Check sheet for the modelled part. Datum: model origin and axes. Units: mm. Face numbers are marked on the shaded views. A direction names the side the tool comes from. Round coordinates to 2 decimals unless told otherwise and drop trailing zeros. Write each loop counter-clockwise with the first axis right and the second up, starting at its lowest first coordinate (ties: lowest second). Pieces come first, ordered by that corner, then holes.
Item 1: Tool access check on the marked faces 1, 2, 3 and 4. Record the directions out of +Z, -Z, +X, -X, +Y, -Y that give a thin tool (end or side, any length) a straight path to the whole face; none if there is none.
Item 2: Cross-section at D-D on y = 4. Enter the section's corners in (x, z).
Item 3: Go/stop test with flat-tipped pins: pin 1 Ø1.5 at (x, z) = (6.5, 2) entering from -Y; pin 2 Ø2 at (x, y) = (8, 0) entering from -Z; pin 3 Ø2 at (x, z) = (10.5, -2.5) entering from -Y; pin 4 Ø4 at (y, z) = (-3.5, 5) entering from +X. Record where each tip stops, or that it passes through.
Item 4: Cross-section at C-C on x = -4.5. Enter the section's corners in (y, z), plus the area to 3 significant figures.
Item 5: Cross-section at B-B on z = 1.5. Enter the section's corners in (x, y).
Item 6: Material ranges on line 1 (X direction, y = -4, z = 3.5); line 2 (X direction, y = -1.5, z = -3.5); line 3 (Z direction, x = -6, y = -1.5), recorded low to high.
from build123d import *

# Parameters (mm, degrees)
SKETCH_1_R          = 3.5
EXTRUDE_1_DEPTH     = 7.3
SKETCH_2_R          = 5
EXTRUDE_2_DEPTH     = 4.1
SKETCH_3_R          = 5
EXTRUDE_3_DEPTH     = 4.1
EXTRUDE_START       = 6
SKETCH_4_R          = 3.5
EXTRUDE_4_DEPTH     = 6
CUT_EXTRUDE_START   = -3.2
CUT_EXTRUDE_1_DEPTH = 3.2


with BuildPart() as part:
    # 草图1 → 凸台-拉伸1 (new body)
    with BuildSketch(Plane(origin=(0, 0, 0), x_dir=(0, 0, -1), z_dir=(1, 0, 0))):
        Circle(SKETCH_1_R)
    extrude(amount=-EXTRUDE_1_DEPTH)

    # 草图2 → 凸台-拉伸2 (add)
    with BuildSketch(Plane(origin=(0, 0, 0), x_dir=(0, 0, -1), z_dir=(1, 0, 0))):
        with Locations((1.49, 0)):
            Circle(SKETCH_2_R)
    extrude(amount=EXTRUDE_2_DEPTH)

    # 草图3 → 凸台-拉伸3 (add)
    with BuildSketch(Plane(origin=(4.1, 0, 0), x_dir=(0, 0, -1), z_dir=(1, 0, 0))):
        with Locations(Location((-1.49, 0, 0), (0, 0, 287.337518018))):
            Circle(SKETCH_3_R)
    extrude(amount=EXTRUDE_3_DEPTH)

    # 草图4 → 凸台-拉伸4 (add)
    with BuildSketch(Plane(origin=(8.2, 0, 0), x_dir=(0, 0, -1), z_dir=(1, 0, 0)).offset(EXTRUDE_START)):
        Circle(SKETCH_4_R)
    extrude(amount=-EXTRUDE_4_DEPTH)

    # 草图7 → 切除-拉伸1 (cut)
    with BuildSketch(Plane.ZY.offset(7.3).offset(CUT_EXTRUDE_START)):
        with BuildLine():
            Line((-2.5, 0), (-3.5, 0))
            ThreePointArc((-3.5, 0), (-3.240370349, -1.322875656), (-2.5, -2.449489743))
            Line((-2.5, -2.449489743), (-2.5, 0))
        make_face()
        with BuildLine():
            ThreePointArc((-2.5, 2.449489743), (-3.240370349, 1.322875656), (-3.5, 0))
            Line((-3.5, 0), (-2.5, 0))
            Line((-2.5, 0), (-2.5, 2.449489743))
        make_face()
        with BuildLine():
            Line((2.5, 0), (2.5, -2.449489743))
            ThreePointArc((2.5, -2.449489743), (3.240370349, -1.322875656), (3.5, 0))
            Line((3.5, 0), (2.5, 0))
        make_face()
        with BuildLine():
            ThreePointArc((3.5, 0), (3.240370349, 1.322875656), (2.5, 2.449489743))
            Line((2.5, 2.449489743), (2.5, 0))
            Line((2.5, 0), (3.5, 0))
        make_face()
    extrude(amount=CUT_EXTRUDE_1_DEPTH, mode=Mode.SUBTRACT)


solid = part.part
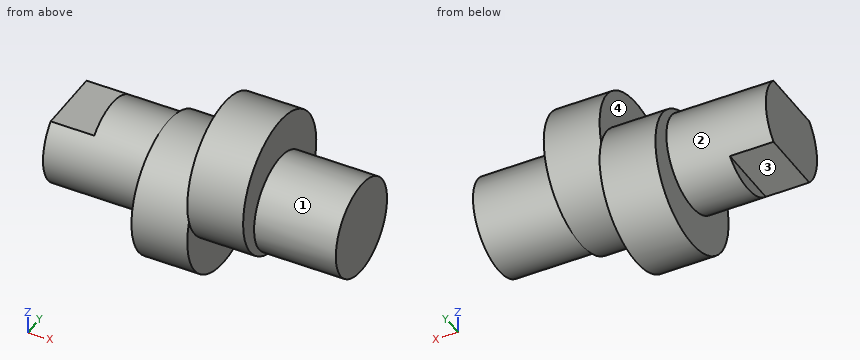
Response values:
1. face 1: +X
1. face 2: -X
1. face 3: -Z, -X, +Y, -Y
1. face 4: +Z, -X
2. outline: (0, -4.49) - (4.1, -4.49) - (4.1, -1.51) - (8.2, -1.51) - (8.2, 4.49) - (4.1, 4.49) - (4.1, 1.51) - (0, 1.51) - close
3. pin 1: stops at y = -5
3. pin 2: stops at z = -3.51
3. pin 3: stops at y = -3.16
3. pin 4: stops at x = 8.2
4. outline: (-2.45, -2.5) - (2.45, -2.5) arc R3.5 ccw to (2.45, 2.5) - (-2.45, 2.5) arc R3.5 ccw to start
4. area: 31.7 mm2
5. outline: (-7.3, -3.16) - (0, -3.16) - (0, -4.01) - (4.1, -4.01) - (4.1, -5) - (8.2, -5) - (8.2, -3.16) - (14.2, -3.16) - (14.2, 3.16) - (8.2, 3.16) - (8.2, 5) - (4.1, 5) - (4.1, 4.01) - (0, 4.01) - (0, 3.16) - (-7.3, 3.16) - close
6. line 1: x = 4.1 to 8.2
6. line 2: x = 0 to 4.1
6. line 3: z = -2.5 to 2.5
